CAD build for the part. Positions are in the model's coordinates, mm. Coordinates: 2 decimals unless noted, no trailing zeros. Order: outer loops, then holes, each group sorted by start corner. A loop starts at its lowest first (then second) coordinate and runs counter-clockwise, first axis right, second up. Notation, with made-up numbers: M 30,12.5 L 72,12.5 A23 ccw 72,33.5 Z; hole C -21.75,-40 d5. An arc over 180 degrees is marked long. One line per item, written item: value.
Autodesk Inventor part; units mm, degrees
ref_plane "Start Plane" through (0, 0, 0) normal (1, 0, 0) x (0, 1, 0)
ref_plane "XZ Plane" through (0, 0, 0) normal (0, 1, 0) x (-1, 0, 0)
ref_plane "XY Plane" through (0, 0, 0) normal (0, 0, 1) x (1, 0, 0)
sketch "Main Sketch" plane through (0, 0, 0) normal (0, 0, 1) x (1, 0, 0)
  line L0 (0, 0) -> (100, 0)
  line L1 (0, 2.5) -> (0, 5)
  line L2 (100, 5) -> (100, 2.5)
  line L3 (0, 5) -> (100, 5)
  line L4 (20, 2.5) -> (20, 0)
  line L5 (0, 2.5) -> (20, 2.5)
  line L6 (80, 2.5) -> (80, 0)
  line L7 (100, 2.5) -> (80, 2.5)
  line L8 (20, 0) -> (80, 0)
  dimension "d3" = 10
  dimension "d4" = 5
  dimension "d5" = 5
revolve "Revolution1" add sketch "Main Sketch" angle 360 about axis through (0, 0, 0) along (1, 0, 0)
equation "\"Length\" = 100"
properties part number "Shaft" material "Steel"
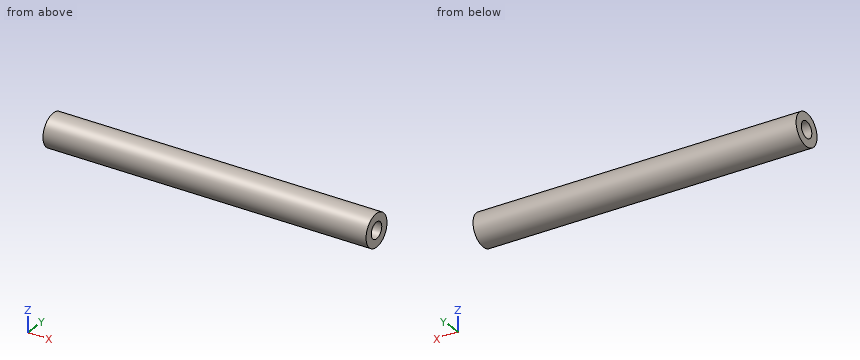
Q1. Drill centre lines: line 1 along Z through (x, y) = (14.25, 0); line 2 along X through (y, z) = (-0.5, 0); line 3 along Y through (x, z) = (90.5, 1.25). Where is each one in solid material? Low to high.
Recorded:
line 1: z = -5 to -2.5, 2.5 to 5
line 2: x = 20 to 80
line 3: y = -4.84 to -2.17, 2.17 to 4.84
Q2. Slice it at D-D (x = 36.5). List the corners of the cut face in (y, z).
Recorded:
outline: C 0,0 d10
Q3. Slice it at B-B (z = 0). List the corners of the cut face in (x, y), plus the area to 3 significant figures.
Recorded:
outline: M 0,-5 L 100,-5 L 100,-2.5 L 80,-2.5 L 80,2.5 L 100,2.5 L 100,5 L 0,5 L 0,2.5 L 20,2.5 L 20,-2.5 L 0,-2.5 Z
area: 800 mm^2
Q4. Slice it at A-A (x = 18.5). List the corners of the cut face in (y, z).
Recorded:
outline: C 0,0 d10; hole C 0,0 d5
Q5. Pin check, flat tips, straight feed: pin 1 Ø1 at (x, y) = (25, 2) entering from -Z; pin 2 Ø1 at (x, y) = (59, -3.5) entering from -Z; pin 3 Ø1.5 at (x, z) = (48, 2) entering from -Y. Stop position of each tip, or through.
Recorded:
pin 1: stops at z = -4.77
pin 2: stops at z = -4
pin 3: stops at y = -4.84
